from build123d import *

# Parameters (mm, degrees)
SKETCH_W               = 104
SKETCH_H               = 50
PAD_DEPTH              = 54
SKETCH001_W            = 42
SKETCH001_H            = 50
POCKET_DEPTH           = 50
SKETCH002_W            = 50
SKETCH002_H            = 50
POCKET001_DEPTH        = 50
POCKET002_DEPTH        = 50.001
SKETCH004_R            = 8.5
POCKET003_DEPTH        = 4.001
SKETCH005_R            = 1.5
POCKET004_DEPTH        = 1
LINEARPATTERN_COUNT    = 4
LINEARPATTERN_PITCH    = 11.333333
SKETCH006_R            = 1.5
POCKET005_DEPTH        = 1
LINEARPATTERN001_COUNT = 4
LINEARPATTERN001_PITCH = 11.666667


with BuildPart() as part:
    # Sketch → Pad (new body)
    with BuildSketch(Plane.XY):
        Rectangle(SKETCH_W, SKETCH_H)
    extrude(amount=PAD_DEPTH)

    # Sketch001 (on Face2 of Pad) → Pocket (cut)
    with BuildSketch(Plane.YZ.offset(52)):
        with Locations((0, 29)):
            Rectangle(SKETCH001_W, SKETCH001_H)
    extrude(amount=-POCKET_DEPTH, mode=Mode.SUBTRACT)

    # Sketch002 (on Face5 of Pocket) → Pocket001 (cut)
    with BuildSketch(Plane.XY.offset(54)):
        with Locations((-27, 0)):
            Rectangle(SKETCH002_W, SKETCH002_H)
    extrude(amount=-POCKET001_DEPTH, mode=Mode.SUBTRACT)

    # Sketch003 (on Face8 of Pocket001) → Pocket002 (cut, through all)
    with BuildSketch(Plane.XZ.offset(25)):
        Polygon((52, 54), (2, 54), (52, 4), align=None)
    extrude(amount=-POCKET002_DEPTH, mode=Mode.SUBTRACT)

    # Sketch004 (on Face11 of Pocket002) → Pocket003 (cut, through all)
    with BuildSketch(Plane.XY.offset(4)):
        with Locations((27, 0)):
            Circle(SKETCH004_R)
    extrude(amount=-POCKET003_DEPTH, mode=Mode.SUBTRACT)

    # Sketch005 (on Face6 of Pocket003) → Pocket004 (cut)
    with BuildSketch(Plane(origin=(-2, 0, 0), x_dir=(0, -1, 0), z_dir=(-1, 0, 0))):
        with Locations((-17, 47)):
            Circle(SKETCH005_R)
        with Locations((-17, 35)):
            Circle(SKETCH005_R)
        with Locations((-17, 23)):
            Circle(SKETCH005_R)
        with Locations((-17, 11)):
            Circle(SKETCH005_R)
    pocket004 = extrude(amount=-POCKET004_DEPTH, mode=Mode.SUBTRACT)

    # LinearPattern: Pocket004 ×4
    with Locations(*[(0, -i * LINEARPATTERN_PITCH, 0) for i in range(1, LINEARPATTERN_COUNT)]):
        add(pocket004, mode=Mode.SUBTRACT)

    # Sketch006 (on Face7 of Pocket003) → Pocket005 (cut)
    with BuildSketch(Plane.XY.offset(4)):
        with Locations((-9, 18)):
            Circle(SKETCH006_R)
        with Locations((-9, 6)):
            Circle(SKETCH006_R)
        with Locations((-9, -6)):
            Circle(SKETCH006_R)
        with Locations((-9, -18)):
            Circle(SKETCH006_R)
    pocket005 = extrude(amount=-POCKET005_DEPTH, mode=Mode.SUBTRACT)

    # LinearPattern001: Pocket005 ×4
    with Locations(*[(-i * LINEARPATTERN001_PITCH, 0, 0) for i in range(1, LINEARPATTERN001_COUNT)]):
        add(pocket005, mode=Mode.SUBTRACT)


solid = part.part
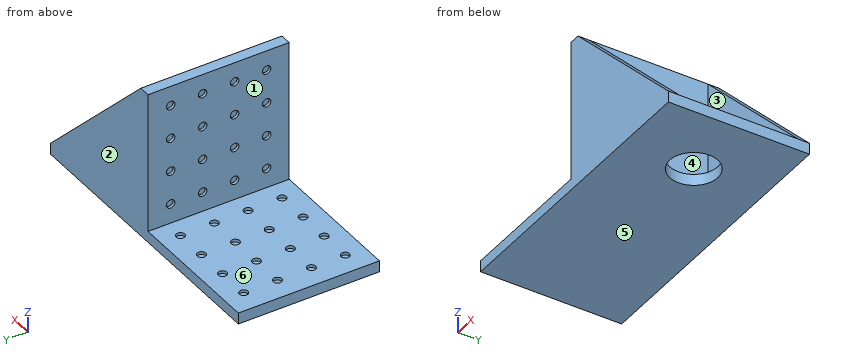
Can you work these out from the model? Positions are in its coordinate system, mm. Face numbers are marked on the shaded views. A direction names the side the tool comes from. Coordinates: 2 decimals unless noted, no trailing zeros. Order: outer loops, then holes, each group sorted by start corner. A loop starts at its lowest first (then second) coordinate and runs counter-clockwise, first axis right, second up. Notation, with made-up numbers: M -0.75,52 L 57.25,52 A32 ccw 57.25,87 Z; hole C 1,9 d3. An arc over 180 degrees is marked long. Answer as CSV lines item,"result".
(1) Suppose I cut it at B-B on x = -9. Please give me the cut outline in (y, z), plus the area to 3 significant figures.
Geometry check:
outline,"M -25,0 L 25,0 L 25,4 L 19.5,4 L 19.5,3 L 16.5,3 L 16.5,4 L 7.5,4 L 7.5,3 L 4.5,3 L 4.5,4 L -4.5,4 L -4.5,3 L -7.5,3 L -7.5,4 L -16.5,4 L -16.5,3 L -19.5,3 L -19.5,4 L -25,4 Z"
area,"188 mm^2"
(2) I'm going to push flat-ended pins straight in: pin 1 (2.5 mm diameter, centred on y = 17, z = 23, fed in from +X); pin 2 (3.5 mm diameter, centred on x = -43.5, y = -6, fed in from +Z); pin 3 (0.9 mm diameter, centred on y = 5, z = 46.5, fed in from -X); pin 4 (5 mm diameter, centred on x = -9, y = 6, fed in from -Z). Where does each tip first touch, or does it pass through?
Geometry check:
pin 1,"x = 2"
pin 2,"z = 4"
pin 3,"x = -1"
pin 4,"z = 0"
(3) Suppose I cut it at D-D on x = 42. Please give me the cut outline in (y, z), plus the area to 3 significant figures.
Geometry check:
outline,"M -25,0 L 25,0 L 25,14 L 21,14 L 21,4 L -21,4 L -21,14 L -25,14 Z"
area,"280 mm^2"
(4) Suppose I cut it at C-C on z = 11. Please give me the cut outline in (x, y), plus the area to 3 significant figures.
Geometry check:
outline,"M -2,-25 L 45,-25 L 45,-21 L 2,-21 L 2,21 L 45,21 L 45,25 L -2,25 L -2,18.5 L -1,18.5 L -1,15.5 L -2,15.5 L -2,7.17 L -1,7.17 L -1,4.17 L -2,4.17 L -2,-4.17 L -1,-4.17 L -1,-7.17 L -2,-7.17 L -2,-15.5 L -1,-15.5 L -1,-18.5 L -2,-18.5 Z"
area,"532 mm^2"
(5) If we mould it in two halves opening along Y, with no side actions, what happens to the marked faces 1, 2 and 3? For each: released by +Y, released by -Y, zero draft, split by the parting line, or undercut.
Geometry check:
face 1,"zero draft"
face 2,"released by +Y"
face 3,"undercut"
(6) Suppose I cut it at A-A on z = 43. Please give me the cut outline in (x, y).
Geometry check:
outline,"M -2,-25 L 13,-25 L 13,-21 L 2,-21 L 2,21 L 13,21 L 13,25 L -2,25 Z"
(7) On a 3-axis mill with a long thin cutter (end or side, diameter ignored), from which of +Z, -Z, +X, -X, +Y, -Y can I reach the whole of each face in a straight line? I mean the marked faces 4, 5 and 6. Say none if no direction works.
Geometry check:
face 4,"+Z, +X"
face 5,"-Z, +X, -X, +Y, -Y"
face 6,"+Z, -X, +Y, -Y"
(8) Please list where these lines run through material, in increasing order: L1, parallel to Z at x = -1.3, y = -17; L2, parallel to X at y = 5.5, z = 45; L3, parallel to Y at x = 23.5, z = 14.5.
Geometry check:
L1,"0 to 9.5, 12.5 to 21.5, 24.5 to 33.5, 36.5 to 45.5, 48.5 to 54"
L2,"-2 to 2"
L3,"-25 to -21, 21 to 25"
